Verification items for the finished model (mm, model axes). Round coordinates to 2 decimals unless told otherwise and drop trailing zeros. Order: outer loops, then holes, each group sorted by start corner. A loop starts at its lowest first (then second) coordinate and runs counter-clockwise, first axis right, second up. Notation, with made-up numbers: (-5, 1.25) -> (37, 1.25) arc R18 cw to (37, 31.25) -> close; hole circle Ø7 at (57, -22). An arc over 180 degrees is marked (long way). Return JSON: item names as keys, results as strings. Group by question number.
Item 1: Sectioned sample at B-B on y = 25.5. Record the cut outline in (x, z) (3 decimals).
Item 2: Draft check along Z on faces 1 (the flat face through (665, 20, 0)), 2 (the flat face through (665, 0, -40)), 3 (the flat face through (668, 29, -81.407)). Enter one of: pulls with the +Z half, pulls with the -Z half, needs draft (parallel to the pull), parting line crosses it, or undercut.
Item 3: Sectioned sample at A-A on x = 781.05. Record the cut outline in (y, z) (3 decimals), plus the area to 3 significant figures.
Item 4: Sectioned sample at C-C on x = 660.5. Record the cut outline in (y, z) (3 decimals), plus the area to 3 significant figures.
Item 5: Depth check by flat-ended pin: pin 1 Ø4 at (x, y) = (612, 46.5) entering from +Z; pin 2 Ø23 at (x, z) = (669, -45) entering from +Y (3 decimals). Enter the tip coordinate at first touch or a pass-through.
Item 6: Sectioned sample at D-D on z = -49. Record the cut outline in (x, y) (3 decimals), plus the area to 3 significant figures.
Item 7: Scan lines: probe 1 along Z at (x, y) = (715, 14.5) (3 decimals); probe 2 along Y at (x, z) = (712.5, -10) (3 decimals); probe 3 along Z at (x, y) = (731.5, 38). Record each from-to range of solid material in increasing order. Write a range as from..to.
```python
from build123d import *

# Parameters (mm, degrees)
SKETCH1_W                    = 787.4
SKETCH1_H                    = 78.232
BOSS_EXTRUDE1_DEPTH          = 3.175
EDGE_FLANGE1_STRIP_W         = 14.224
EDGE_FLANGE1_STRIP_H         = 3.175
EDGE_FLANGE1_STRIP_CUT_DEPTH = 787.4
EDGE_FLANGE1_DEPTH           = 787.4
EDGE_FLANGE2_STRIP_W         = 14.224
EDGE_FLANGE2_STRIP_H         = 3.175
EDGE_FLANGE2_STRIP_CUT_DEPTH = 787.4
EDGE_FLANGE2_DEPTH           = 787.4
SKETCH9_R                    = 2.667
CUT_EXTRUDE1_DEPTH           = 794.767078776
CHAMFER1_SIZE                = 3.175
LPATTERN1_COUNT              = 62
LPATTERN1_PITCH              = 12.7
SKETCH12_R                   = 1.27
CUT_EXTRUDE4_DEPTH           = 794.225377588
SKETCH14_R                   = 2.667
CUT_EXTRUDE6_DEPTH           = 5.08
LPATTERN4_COUNT              = 62
LPATTERN4_PITCH              = 12.7
SKETCH15_W                   = 546.1
SKETCH15_H                   = 84.582
CUT_EXTRUDE7_DEPTH           = 794.435038471


# Sheet-metal steps are written as plain solids
with BuildPart() as part:
    # Sketch1 → Boss-Extrude1 (new body)
    with BuildSketch(Plane(origin=(0, 0, 0), x_dir=(1, 0, 0), z_dir=(0, 1, 0))):
        with Locations((393.7, 39.116)):
            Rectangle(SKETCH1_W, SKETCH1_H)
    extrude(amount=BOSS_EXTRUDE1_DEPTH)

    # Edge-Flange1 strip (across the edge) → Edge-Flange1 strip cut (cut)
    with BuildSketch(Plane(origin=(787.4, 3.175, -78.232), x_dir=(0, 0, 1), z_dir=(-1, 0, 0))):
        with Locations((-6.35, -1.5875)):
            Rectangle(EDGE_FLANGE1_STRIP_W, EDGE_FLANGE1_STRIP_H)
    extrude(amount=EDGE_FLANGE1_STRIP_CUT_DEPTH, mode=Mode.SUBTRACT)

    # Edge-Flange1 section (across the edge) → Edge-Flange1 (add)
    with BuildSketch(Plane(origin=(787.4, 3.175, -78.232), x_dir=(0, 0, 1), z_dir=(-1, 0, 0))):
        with BuildLine():
            Line((-3.175, 0.762), (-3.175, 50.8))
            Line((-3.175, 50.8), (0, 50.8))
            Line((0, 50.8), (0, 0.762))
            ThreePointArc((0, 0.762), (0.223184633, 0.223184633), (0.762, 0))
            Line((0.762, 0), (0.762, -3.175))
            ThreePointArc((0.762, -3.175), (-2.021879398, -2.021879398), (-3.175, 0.762))
        make_face()
    extrude(amount=EDGE_FLANGE1_DEPTH)

    # Edge-Flange2 strip (across the edge) → Edge-Flange2 strip cut (cut)
    with BuildSketch(Plane(origin=(0, 3.175, 0), x_dir=(0, 0, -1), z_dir=(1, 0, 0))):
        with Locations((-6.35, -1.5875)):
            Rectangle(EDGE_FLANGE2_STRIP_W, EDGE_FLANGE2_STRIP_H)
    extrude(amount=EDGE_FLANGE2_STRIP_CUT_DEPTH, mode=Mode.SUBTRACT)

    # Edge-Flange2 section (across the edge) → Edge-Flange2 (add)
    with BuildSketch(Plane(origin=(0, 3.175, 0), x_dir=(0, 0, -1), z_dir=(1, 0, 0))):
        with BuildLine():
            Line((-3.175, 0.762), (-3.175, 31.75))
            Line((-3.175, 31.75), (0, 31.75))
            Line((0, 31.75), (0, 0.762))
            ThreePointArc((0, 0.762), (0.223184633, 0.223184633), (0.762, 0))
            Line((0.762, 0), (0.762, -3.175))
            ThreePointArc((0.762, -3.175), (-2.021879398, -2.021879398), (-3.175, 0.762))
        make_face()
    extrude(amount=EDGE_FLANGE2_DEPTH)

    # Sketch9 → Cut-Extrude1 (cut, through all)
    with BuildSketch(Plane.XY.offset(3.175)):
        with Locations((781.05, 16.637)):
            Circle(SKETCH9_R)
    cut_extrude1 = extrude(amount=-CUT_EXTRUDE1_DEPTH, mode=Mode.SUBTRACT)

    # Chamfer1
    chamfer1_edges = [part.edges().sort_by_distance(p)[0] for p in [
        (787.4, 53.975, -79.8195),
        (0, 53.975, -79.8195),
        (0, 34.925, 1.5875),
        (787.4, 34.925, 1.5875),
    ]]
    chamfer(chamfer1_edges, length=CHAMFER1_SIZE)

    # LPattern1: Cut-Extrude1 ×62
    with Locations(*[(-i * LPATTERN1_PITCH, 0, 0) for i in range(1, LPATTERN1_COUNT)]):
        add(cut_extrude1, mode=Mode.SUBTRACT)

    # Sketch12 → Cut-Extrude4 (cut, through all)
    with BuildSketch(Plane(origin=(0, 3.175, 0), x_dir=(1, 0, 0), z_dir=(0, 1, 0))):
        with Locations(Location((101.6, 72.39, 0), (0, 0, 270))):
            Circle(SKETCH12_R)
        with Locations(Location((215.9, 72.39, 0), (0, 0, 270))):
            Circle(SKETCH12_R)
        with Locations(Location((215.9, 5.842, 0), (0, 0, 270))):
            Circle(SKETCH12_R)
        with Locations(Location((101.6, 5.842, 0), (0, 0, 270))):
            Circle(SKETCH12_R)
    extrude(amount=-CUT_EXTRUDE4_DEPTH, mode=Mode.SUBTRACT)

    # Sketch14 → Cut-Extrude6 (cut)
    with BuildSketch(Plane(origin=(0, 0, -81.407), x_dir=(-1, 0, 0), z_dir=(0, 0, -1))):
        with Locations(Location((-781.05, 42.037, 0), (0, 0, 90))):
            Circle(SKETCH14_R)
    cut_extrude6 = extrude(amount=-CUT_EXTRUDE6_DEPTH, mode=Mode.SUBTRACT)

    # LPattern4: Cut-Extrude6 ×62
    with Locations(*[(-i * LPATTERN4_PITCH, 0, 0) for i in range(1, LPATTERN4_COUNT)]):
        add(cut_extrude6, mode=Mode.SUBTRACT)

    # Sketch15 → Cut-Extrude7 (cut, through all)
    with BuildSketch(Plane(origin=(0, 53.975, 0), x_dir=(1, 0, 0), z_dir=(0, 1, 0))):
        with Locations((273.05, 39.116)):
            Rectangle(SKETCH15_W, SKETCH15_H)
    extrude(amount=-CUT_EXTRUDE7_DEPTH, mode=Mode.SUBTRACT)


solid = part.part
```
Recorded:
{
 "1": {"outline": "(546.1, -81.407) -> (787.4, -81.407) -> (787.4, -78.232) -> (546.1, -78.232) -> close; (546.1, 0) -> (787.4, 0) -> (787.4, 3.175) -> (546.1, 3.175) -> close"},
 "2": {"face 1": "undercut", "face 2": "needs draft", "face 3": "pulls with the -Z half"},
 "3": {"outline": "(0, -77.47) arc R3.937 ccw to (3.937, -81.407) -> (13.97, -81.407) -> (13.97, -78.232) -> (3.937, -78.232) arc R0.762 cw to (3.175, -77.47) -> (3.175, -0.762) arc R0.762 cw to (3.937, 0) -> (13.97, 0) -> (13.97, 3.175) -> (3.937, 3.175) arc R3.937 ccw to (0, -0.762) -> close; (19.304, -81.407) -> (39.37, -81.407) -> (39.37, -78.232) -> (19.304, -78.232) -> close; (19.304, 0) -> (34.925, 0) -> (34.925, 3.175) -> (19.304, 3.175) -> close; (44.704, -81.407) -> (53.975, -81.407) -> (53.975, -78.232) -> (44.704, -78.232) -> close", "area": "473 mm²"},
 "4": {"outline": "(0, -77.47) arc R3.937 ccw to (3.937, -81.407) -> (53.975, -81.407) -> (53.975, -78.232) -> (3.937, -78.232) arc R0.762 cw to (3.175, -77.47) -> (3.175, -0.762) arc R0.762 cw to (3.937, 0) -> (34.925, 0) -> (34.925, 3.175) -> (3.937, 3.175) arc R3.937 ccw to (0, -0.762) -> close", "area": "524 mm²"},
 "5": {"pin 1": "z = -78.23", "pin 2": "y = 3.175"},
 "6": {"outline": "(546.1, 0) -> (787.4, 0) -> (787.4, 3.175) -> (546.1, 3.175) -> close", "area": "766 mm²"},
 "7": {"probe 1": "-81.407..-78.232, 0..3.175", "probe 2": "0..3.175", "probe 3": "-81.41..-78.23"}
}
